The listing builds one solid part. Answer for the finished solid, in the listing's coordinates (mm). Face numbers are marked on the shaded views. A direction names the side the tool comes from. Coordinates: 2 decimals unless noted, no trailing zeros. Loops run counter-clockwise (first coordinate to the right, second up) from the corner with the lowest first, then second, coordinate; pieces in that order, holes last. Notation, with made-up numbers: (8.5, -22.75) - (49.5, -22.75) arc R28 cw to (49.5, 11.25) - close; hole circle Ø5 at (-0.5, -27). An arc over 180 degrees is marked (long way). Write each question's results on one line, items separated by ' | '. Start each with the question number.
(1) Consider line 1 (Y direction, x = 63.7, z = 0.65); line 2 (Y direction, x = 106, z = -5.5); line 3 (Z direction, x = 129, y = 63). Determine where each line is inside the solid, lowest interval first. Write a range as from..to.
(2) Find section B-B on z = 23. Determine the outline of the cut face in (x, y).
(3) Find section A-A on y = 12.5. State how many separate pieces and enclosed holes the cut face has, then the cut area to 3 significant figures.
(4) Given pin 1 Ø2.5 at (x, y) = (127.7, 115) entering from +Z; pin 2 Ø0.5 at (x, z) = (11, 7) entering from +Y; pin 3 Ø3 at (x, y) = (84, 61) entering from -Z; pin 4 Ø8 at (x, z) = (71.5, -10.5) entering from +Y, each flat-ended and moving along its own axis, determine where each tip first touches the part or whether it passes through.
(5) Find section C-C on x = 17. Determine the outline of the cut face in (y, z).
(6) For the marked faces 1, 2 and 3, determine the directions among +Z, -Z, +X, -X, +Y, -Y from which every point of the face is accessible in a straight line to the end or side of a thin tool.
(7) Find section D-D on y = 91. Determine the outline of the cut face in (x, z), then the cut area to 4 significant figures.
(8) Determine the mould class of the marked faces 4, 5 and 6 for opening direction X: released by +X, released by -X, zero draft, split by the parting line, or undercut.
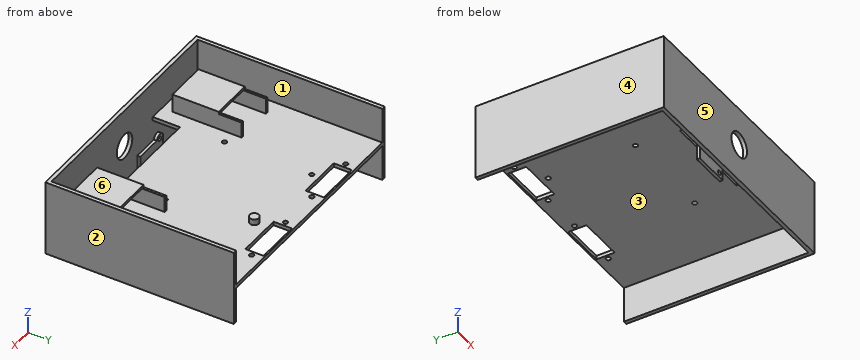
from build123d import *

# Parameters (mm, degrees)
SKETCH1_W           = 155.4
SKETCH1_H           = 122
SKETCH1_R           = 1.5
SKETCH1_W_2         = 30
SKETCH1_H_2         = 12
BOSS_EXTRUDE1_DEPTH = 2.5
SKETCH1_5_R         = 3
BOSS_EXTRUDE2_DEPTH = 6.5
BOSS_EXTRUDE3_DEPTH = 13
SKETCH2_W           = 27.7
SKETCH2_H           = 30.6
BOSS_EXTRUDE4_DEPTH = 1.6
SKETCH3_W           = 155.4
SKETCH3_H           = 50
SKETCH3_R           = 8.25
BOSS_EXTRUDE5_DEPTH = 2.5
SKETCH4_W           = 60
SKETCH4_H           = 18
CUT_EXTRUDE1_DEPTH  = 10
SKETCH6_R           = 1.5
BOSS_EXTRUDE6_DEPTH = 2
SKETCH7_W           = 50
SKETCH7_H           = 124.5
BOSS_EXTRUDE7_DEPTH = 2.5
SKETCH8_W           = 50
SKETCH8_H           = 124.5
BOSS_EXTRUDE8_DEPTH = 2.5


with BuildPart() as part:
    # Sketch1 → Boss-Extrude1 (new body)
    with BuildSketch(Plane.XY):
        with Locations((77.7, 61)):
            Rectangle(SKETCH1_W, SKETCH1_H)
        with Locations((46.223, 104.1)):
            Circle(SKETCH1_R, mode=Mode.SUBTRACT)
        with Locations((46.2, 46.5)):
            Circle(SKETCH1_R, mode=Mode.SUBTRACT)
        with Locations((109.2, 46.5)):
            Circle(SKETCH1_R, mode=Mode.SUBTRACT)
        with Locations((63.7, 115)):
            Circle(SKETCH1_R, mode=Mode.SUBTRACT)
        with Locations((27.7, 115)):
            Circle(SKETCH1_R, mode=Mode.SUBTRACT)
        with Locations((91.7, 115)):
            Circle(SKETCH1_R, mode=Mode.SUBTRACT)
        with Locations((127.7, 115)):
            Circle(SKETCH1_R, mode=Mode.SUBTRACT)
        with Locations((45.7, 115)):
            Rectangle(SKETCH1_W_2, SKETCH1_H_2, mode=Mode.SUBTRACT)
        with Locations((109.7, 115)):
            Rectangle(SKETCH1_W_2, SKETCH1_H_2, mode=Mode.SUBTRACT)
    extrude(amount=BOSS_EXTRUDE1_DEPTH)

    # Sketch1_5 → Boss-Extrude2 (add)
    with BuildSketch(Plane.XY):
        with Locations((100.7, 100)):
            Circle(SKETCH1_5_R)
    extrude(amount=BOSS_EXTRUDE2_DEPTH)

    # Sketch1_6 → Boss-Extrude3 (add)
    with BuildSketch(Plane.XY):
        Polygon((145.4, 52.4), (145.4, 6.8), (117.7, 6.8), (117.7, 52.4), (119.3, 52.4), (119.3, 8.4), (143.8, 8.4), (143.8, 52.4), align=None)
        Polygon((10, 6.8), (37.7, 6.8), (37.7, 52.4), (36.1, 52.4), (36.1, 8.4), (11.6, 8.4), (11.6, 52.4), (10, 52.4), align=None)
    extrude(amount=BOSS_EXTRUDE3_DEPTH)

    # Sketch2 → Boss-Extrude4 (add)
    with BuildSketch(Plane.XY.offset(13)):
        with Locations((23.85, 22.1)):
            Rectangle(SKETCH2_W, SKETCH2_H)
        with Locations((131.55, 22.1)):
            Rectangle(SKETCH2_W, SKETCH2_H)
    extrude(amount=BOSS_EXTRUDE4_DEPTH)

    # Sketch3 → Boss-Extrude5 (add)
    with BuildSketch(Plane.XZ):
        with Locations((77.7, 1.25)):
            Rectangle(SKETCH3_W, SKETCH3_H)
        with Locations((77.7, 1.25)):
            Circle(SKETCH3_R, mode=Mode.SUBTRACT)
    extrude(amount=BOSS_EXTRUDE5_DEPTH)

    # Sketch4 → Cut-Extrude1 (cut)
    with BuildSketch(Plane.XY.offset(2.5)):
        with Locations((77.7, 9)):
            Rectangle(SKETCH4_W, SKETCH4_H)
    extrude(amount=-CUT_EXTRUDE1_DEPTH, mode=Mode.SUBTRACT)

    # Sketch6 → Boss-Extrude6 (add)
    with BuildSketch(Plane.XZ.offset(-18)):
        with BuildLine():
            Line((89.85, 8.759024603), (72.353800708, 8.759024603))
            ThreePointArc((72.353800708, 8.759024603), (68.592638026, 11.375865762), (65.55, 7.95))
            Line((65.55, 7.95), (65.55, -8.65))
            Line((65.55, -8.65), (89.85, -8.65))
            Line((89.85, -8.65), (89.85, 8.759024603))
        make_face()
        with Locations((69, 7.95)):
            Circle(SKETCH6_R, mode=Mode.SUBTRACT)
        with Locations((86.4, -5.45)):
            Circle(SKETCH6_R, mode=Mode.SUBTRACT)
    extrude(amount=BOSS_EXTRUDE6_DEPTH)

    # Sketch7 → Boss-Extrude7 (add)
    with BuildSketch(Plane(origin=(155.4, 0, 0), x_dir=(0, 0, -1), z_dir=(1, 0, 0))):
        with Locations((-1.25, 59.75)):
            Rectangle(SKETCH7_W, SKETCH7_H)
    extrude(amount=BOSS_EXTRUDE7_DEPTH)

    # Sketch8 → Boss-Extrude8 (add)
    with BuildSketch(Plane.ZY):
        with Locations((1.25, 59.75)):
            Rectangle(SKETCH8_W, SKETCH8_H)
    extrude(amount=BOSS_EXTRUDE8_DEPTH)


solid = part.part
Values:
1) line 1: y = -2.5..0, 18..113.5, 116.5..122 | line 2: y = -2.5..0 | line 3: z = 0..2.5
2) outline: (-2.5, -2.5) - (157.9, -2.5) - (157.9, 122) - (155.4, 122) - (155.4, 0) - (0, 0) - (0, 122) - (-2.5, 122) - close
3) separate pieces: 2 | enclosed holes: 2 | area: 644 mm²
4) pin 1: passes through | pin 2: stops at y = 52.4 | pin 3: stops at z = 0 | pin 4: stops at y = 18
5) outline: (-2.5, -23.75) - (0, -23.75) - (0, 0) - (122, 0) - (122, 2.5) - (8.4, 2.5) - (8.4, 13) - (37.4, 13) - (37.4, 14.6) - (6.8, 14.6) - (6.8, 2.5) - (0, 2.5) - (0, 26.25) - (-2.5, 26.25) - close
6) face 1: +Z, +Y | face 2: +Z, -Z, +X, +Y, -Y | face 3: -Z, +Y
7) outline: (-2.5, -23.75) - (0, -23.75) - (0, 0) - (155.4, 0) - (155.4, -23.75) - (157.9, -23.75) - (157.9, 26.25) - (155.4, 26.25) - (155.4, 2.5) - (0, 2.5) - (0, 26.25) - (-2.5, 26.25) - close | area: 638.5 mm²
8) face 4: released by -X | face 5: zero draft | face 6: undercut
